The listing builds one solid part. Answer for the finished solid, in the listing's coordinates (mm). Face numbers are marked on the shaded views. A direction names the side the tool comes from. Coordinates: 2 decimals unless noted, no trailing zeros. Write each loop counter-clockwise with the first axis right and the second up, starting at its lowest first coordinate (ties: lowest second). Pieces come first, ordered by that corner, then holes. Notation, with made-up numbers: M -14.75,77 L -4.75,77 A13 ccw -4.75,82 Z; hole C 81,74 d1. An arc over 180 degrees is marked long. Put each result on its own line as item: value. Start each with the question number.
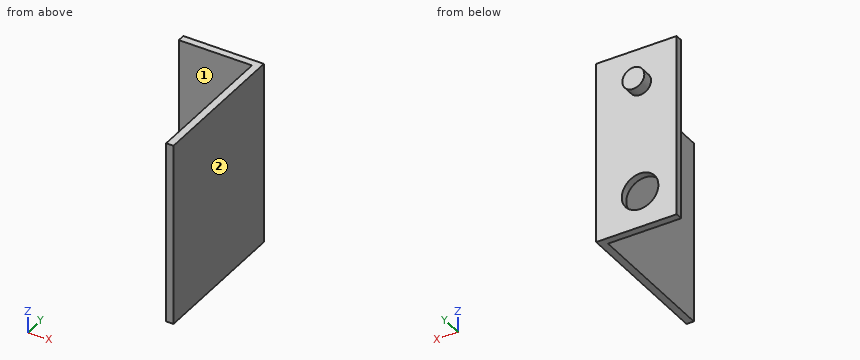
```python
from build123d import *

# Parameters (mm, degrees)
SALIENTE_EXTRUIR1_DEPTH = 50
CORTAR_EXTRUIR1_REACH   = 69.705
CROQUIS2_R              = 5
CROQUIS3_R              = 3
SALIENTE_EXTRUIR2_DEPTH = 3


with BuildPart() as part:
    # Croquis1 → Saliente-Extruir1 (new body)
    with BuildSketch(Plane.XY):
        Polygon((0, 0), (0, 2), (22, 2), (22, -38), (20, -38), (20, 0), align=None)
    extrude(amount=SALIENTE_EXTRUIR1_DEPTH)

    # Croquis2 → Cortar-Extruir1 (cut, up to next)
    with BuildSketch(Plane(origin=(0, 2, 0), x_dir=(1, 0, 0), z_dir=(0, 1, 0)), mode=Mode.PRIVATE) as cortar_extruir1_sk1:
        with Locations(Location((10, -10, 0), (0, 0, 270))):
            Circle(CROQUIS2_R)
    cortar_extruir1_tool1 = extrude(cortar_extruir1_sk1.sketch, amount=-CORTAR_EXTRUIR1_REACH, mode=Mode.PRIVATE) & part.part
    add(cortar_extruir1_tool1.solids().sort_by_distance((10, 2, 10))[0], mode=Mode.SUBTRACT)

    # Croquis3 → Saliente-Extruir2 (add)
    with BuildSketch(Plane(origin=(0, 2, 0), x_dir=(1, 0, 0), z_dir=(0, 1, 0))):
        with Locations(Location((10, -40, 0), (0, 0, 90))):
            Circle(CROQUIS3_R)
    extrude(amount=SALIENTE_EXTRUIR2_DEPTH)


solid = part.part
```
1) A cutting plane is placed at B-B on x = 14. Write down the section's boundary in (y, z), then the cut area to 3 significant figures.
2) Given pin 1 Ø1.5 at (y, z) = (-32.5, 25) entering from -X; pin 2 Ø6 at (x, z) = (10, 36) entering from -Y; pin 3 Ø9 at (x, z) = (10, 10) entering from +Y, each flat-ended and moving along its own axis, determine where each tip first touches the part or whether it passes through.
3) A cutting plane is placed at C-C on x = 10. Write down the section's boundary in (y, z).
4) A cutting plane is placed at A-A on z = 10. Write down the section's boundary in (x, y), then the cut area to 4 significant figures.
5) A cutting plane is placed at D-D on z = 22. Write down the section's boundary in (x, y).
6) Straight lines are drawn through the part: probe 1 along X at (y, z) = (1, 10); probe 2 along Y at (x, z) = (1.75, 12); probe 3 along X at (y, z) = (-36, 10). For each, find the intervals that lie inside material, in ascending order.
7) For the marked faces 1 and 2, determine the directions among +Z, -Z, +X, -X, +Y, -Y from which every point of the face is accessible in a straight line to the end or side of a thin tool.
Answers follow:
1. outline: M 0,0 L 2,0 L 2,7 L 0,7 Z; M 0,13 L 2,13 L 2,50 L 0,50 Z
1. area: 88.0 mm²
2. pin 1: stops at x = 20
2. pin 2: stops at y = 0
2. pin 3: passes through
3. outline: M 0,0 L 2,0 L 2,5 L 0,5 Z; M 0,15 L 2,15 L 2,37 L 5,37 L 5,43 L 2,43 L 2,50 L 0,50 Z
4. outline: M 0,0 L 5,0 L 5,2 L 0,2 Z; M 15,0 L 20,0 L 20,-38 L 22,-38 L 22,2 L 15,2 Z
4. area: 100.0 mm²
5. outline: M 0,0 L 20,0 L 20,-38 L 22,-38 L 22,2 L 0,2 Z
6. probe 1: x = 0 to 5, 15 to 22
6. probe 2: y = 0 to 2
6. probe 3: x = 20 to 22
7. face 1: +Z, -Z, -X, -Y
7. face 2: +Z, -Z, +X, +Y, -Y
